Design review of the part built by this model. Coordinates are the model's own, in mm. Give positions to 0.01 mm unless a question says otherwise; leave off trailing zeros. Loops run counter-clockwise (first coordinate to the right, second up) from the corner with the lowest first, then second, coordinate; pieces in that order, holes last. Notation, with made-up numbers: (49, 45.5) - (57, 45.5) arc R13 cw to (57, 61.5) - close; hole circle Ø11 at (-30.5, 69). An arc over 180 degrees is marked (long way). One line per item, written item: value. Start each with the question number.
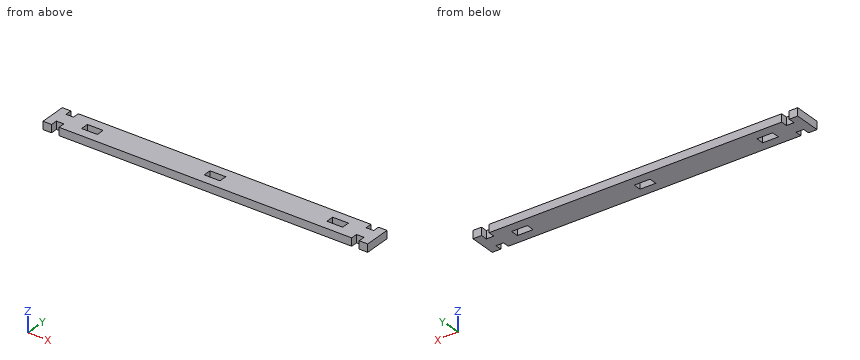
```python
from build123d import *

# Parameters (mm, degrees)
SKETCH1_W           = 12
SKETCH1_H           = 6
BOSS_EXTRUDE1_DEPTH = 6


with BuildPart() as part:
    # Sketch1 → Boss-Extrude1 (new body)
    with BuildSketch(Plane.XY):
        Polygon((-123.5, 10), (-123.5, -10), (-117, -10), (-117, -5), (-111.3, -5), (-111.3, -10), (111.3, -10), (111.3, -5), (117, -5), (117, -10), (123.5, -10), (123.5, 10), (117, 10), (117, 5), (111.3, 5), (111.3, 10), (-111.3, 10), (-111.3, 5), (-117, 5), (-117, 10), align=None)
        with Locations((93.3, 0)):
            Rectangle(SKETCH1_W, SKETCH1_H, mode=Mode.SUBTRACT)
        with Locations((-93.3, 0)):
            Rectangle(SKETCH1_W, SKETCH1_H, mode=Mode.SUBTRACT)
        Rectangle(SKETCH1_W, SKETCH1_H, mode=Mode.SUBTRACT)
    extrude(amount=-BOSS_EXTRUDE1_DEPTH)


solid = part.part
```
(1) To check wall thickness, follow L1, parallel to X at y = -0.5, z = -3.7; L2, parallel to X at y = 8, z = -3.9; L3, parallel to Y at x = -94.5, z = -0.95. State the ranges of each line that lie inside material, in increasing order. Write a range as from..to.
(2) Take a section at B-B on y = -1. State the section outline as (x, z) points, and give its area (3 significant figures).
(3) Take a section at A-A on x = -90.5. State the section outline as (y, z) points, and give its area (3 significant figures).
(4) For pin 1 Ø5 at (x, y) = (-23.5, 5.5) entering from +Z; pin 2 Ø1.7 at (x, z) = (113.5, -3.5) entering from +Y; pin 3 Ø3 at (x, z) = (-113.5, -3.5) entering from -Y, all flat-tipped, find the tip position at first contact; note any pin that passes through.
(5) Take a section at C-C on z = -2.55. State how many separate pieces and enclosed holes the cut face has, and give its area (3 significant figures).
Here are the results:
1. L1: -123.5..-99.3, -87.3..-6, 6..87.3, 99.3..123.5
1. L2: -123.5..-117, -111.3..111.3, 117..123.5
1. L3: -10..-3, 3..10
2. outline: (-123.5, -6) - (-99.3, -6) - (-99.3, 0) - (-123.5, 0) - close; (-87.3, -6) - (-6, -6) - (-6, 0) - (-87.3, 0) - close; (6, -6) - (87.3, -6) - (87.3, 0) - (6, 0) - close; (99.3, -6) - (123.5, -6) - (123.5, 0) - (99.3, 0) - close
2. area: 1,270 mm²
3. outline: (-10, -6) - (-3, -6) - (-3, 0) - (-10, 0) - close; (3, -6) - (10, -6) - (10, 0) - (3, 0) - close
3. area: 84.0 mm²
4. pin 1: z = 0
4. pin 2: y = 5
4. pin 3: y = -5
5. separate pieces: 1
5. enclosed holes: 3
5. area: 4,610 mm²
